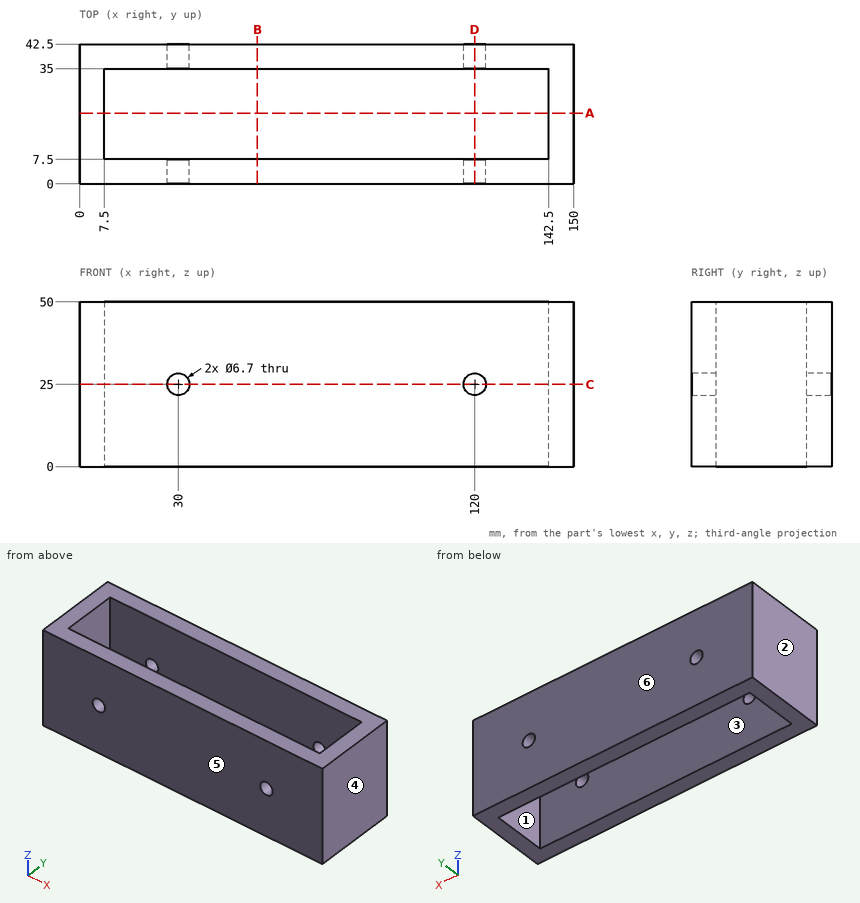
The drawing under review shows one solid part. Ordinate dimensions are in mm from its lowest x, y, z. A direction names the side the tool comes from. Coordinates: 2 decimals unless noted, no trailing zeros. Write each loop counter-clockwise with the first axis right and the second up, starting at its lowest first coordinate (ties: lowest second). Pieces come first, ordered by that corner, then holes. Notation, with made-up numbers: (-8.75, 26.25) -> (21.25, 26.25) arc R23 ccw to (21.25, 43.25) -> close; hole circle Ø5 at (-4.75, 54). An arc over 180 degrees is marked (long way). One line per item, written item: value. Start each with the question number.
Q1. To check wall thickness, follow probe 1 along X at (y, z) = (5, 25); probe 2 along Y at (x, z) = (55, 3); probe 3 along X at (y, z) = (5, 27). State the ranges of each line that lie inside material, in increasing order.
Q2. Add section A-A, the plane y = 21.5. Give the boundary of the cut face in (x, z).
Q3. Add section C-C, the plane z = 25. Give the boundary of the cut face in (x, y).
Q4. Add section B-B, the plane x = 54. Give the boundary of the cut face in (y, z).
Q5. The part is to be moulded in two halves that separate along Y. For the marked faces 3, 4, 5 and 6, say which applies: +Y half, -Y half, draft (parallel to the pull), parting line (faces both ways), or undercut.
Q6. For the marked faces 1 and 2, list the 3-axis set-ups (+Z, -Z, +X, -X, +Y, -Y) from which the entire face can be reached by the end or side of a thin tool; tool diameter is ignored.
Q7. Clearance check with a flat-ended pin moving along its axis: P1, Ø10.5, axis at x = 120, z = 25, coming from the +Y side. State where the tip first meets the part, or that it passes through.
Q8. Add section D-D, the plane x = 120. Give the boundary of the cut face in (y, z).
Response:
1. probe 1: 0 to 26.65, 33.35 to 116.65, 123.35 to 150
1. probe 2: 0 to 7.5, 35 to 42.5
1. probe 3: 0 to 27.31, 32.69 to 117.31, 122.69 to 150
2. outline: (0, 0) -> (7.5, 0) -> (7.5, 50) -> (0, 50) -> close; (142.5, 0) -> (150, 0) -> (150, 50) -> (142.5, 50) -> close
3. outline: (0, 0) -> (26.65, 0) -> (26.65, 7.5) -> (7.5, 7.5) -> (7.5, 35) -> (26.65, 35) -> (26.65, 42.5) -> (0, 42.5) -> close; (33.35, 0) -> (116.65, 0) -> (116.65, 7.5) -> (33.35, 7.5) -> close; (33.35, 35) -> (116.65, 35) -> (116.65, 42.5) -> (33.35, 42.5) -> close; (123.35, 0) -> (150, 0) -> (150, 42.5) -> (123.35, 42.5) -> (123.35, 35) -> (142.5, 35) -> (142.5, 7.5) -> (123.35, 7.5) -> close
4. outline: (0, 0) -> (7.5, 0) -> (7.5, 50) -> (0, 50) -> close; (35, 0) -> (42.5, 0) -> (42.5, 50) -> (35, 50) -> close
5. face 3: undercut
5. face 4: draft
5. face 5: -Y half
5. face 6: +Y half
6. face 1: +Z, -Z
6. face 2: +Z, -Z, -X, +Y, -Y
7. P1: y = 42.5
8. outline: (0, 0) -> (7.5, 0) -> (7.5, 21.65) -> (0, 21.65) -> close; (0, 28.35) -> (7.5, 28.35) -> (7.5, 50) -> (0, 50) -> close; (35, 0) -> (42.5, 0) -> (42.5, 21.65) -> (35, 21.65) -> close; (35, 28.35) -> (42.5, 28.35) -> (42.5, 50) -> (35, 50) -> close
